from build123d import *

# Parameters (mm, degrees)
SKETCH1_W               = 20
SKETCH1_H               = 20
BOSS_EXTRUDE1_DEPTH     = 5
SKETCH2_W               = 20
SKETCH2_H               = 3
BOSS_EXTRUDE2_DEPTH     = 20
CUT_EXTRUDE1_DEPTH      = 25.494897428
CUT_EXTRUDE1_DEPTH_BACK = 25.494897428
SKETCH3_R               = 2.6
BOSS_EXTRUDE3_DEPTH     = 2
BOSS_EXTRUDE4_DEPTH     = 2
SKETCH6_W               = 2
SKETCH6_H               = 3
SKETCH6_W_2             = 4
BOSS_EXTRUDE5_DEPTH     = 0.8
SKETCH9_W               = 20
SKETCH9_H               = 3
BOSS_EXTRUDE8_DEPTH     = 45
BOSS_EXTRUDE9_DEPTH     = 20
SKETCH13_W              = 20
SKETCH13_H              = 3
BOSS_EXTRUDE12_DEPTH    = 80
SKETCH16_W              = 3
SKETCH16_H              = 45
CUT_EXTRUDE3_DEPTH      = 80
SKETCH22_W              = 20
SKETCH22_H              = 80
BOSS_EXTRUDE15_DEPTH    = 3
BOSS_EXTRUDE16_DEPTH    = 2
BOSS_EXTRUDE17_DEPTH    = 2
FILLET2_R               = 3
SKETCH26_R              = 2.4
CUT_EXTRUDE5_DEPTH      = 9


with BuildPart() as part:
    # Sketch1 → Boss-Extrude1 (new body)
    with BuildSketch(Plane(origin=(0, 0, 0), x_dir=(1, 0, 0), z_dir=(0, 1, 0))):
        Rectangle(SKETCH1_W, SKETCH1_H)
    extrude(amount=BOSS_EXTRUDE1_DEPTH)

    # Sketch2 → Boss-Extrude2 (add)
    with BuildSketch(Plane(origin=(0, 5, 0), x_dir=(1, 0, 0), z_dir=(0, 1, 0))):
        with Locations((0, 8.5)):
            Rectangle(SKETCH2_W, SKETCH2_H)
    extrude(amount=BOSS_EXTRUDE2_DEPTH)

    # Sketch3 → Cut-Extrude1 (cut, two sides: drawn at the far end of the back side and taken through both)
    with BuildSketch(Plane(origin=(0, 5, 0), x_dir=(1, 0, 0), z_dir=(0, 1, 0)).offset(-CUT_EXTRUDE1_DEPTH_BACK)):
        with Locations(Location((0, -1.5, 0), (0, 0, 270))):
            Circle(SKETCH3_R)
    extrude(amount=CUT_EXTRUDE1_DEPTH + CUT_EXTRUDE1_DEPTH_BACK, mode=Mode.SUBTRACT)

    # Sketch4 → Boss-Extrude3 (add)
    with BuildSketch(Plane.ZY.offset(10)):
        Polygon((-7, 25), (10, 5), (-7, 5), align=None)
    extrude(amount=-BOSS_EXTRUDE3_DEPTH)

    # Sketch5 → Boss-Extrude4 (add)
    with BuildSketch(Plane(origin=(10, 0, 0), x_dir=(0, 0, -1), z_dir=(1, 0, 0))):
        Polygon((7, 25), (-10, 5), (7, 5), align=None)
    extrude(amount=-BOSS_EXTRUDE4_DEPTH)

    # Sketch6 → Boss-Extrude5 (add)
    with BuildSketch(Plane(origin=(0, 0, 0), x_dir=(-1, 0, 0), z_dir=(0, -1, 0))):
        with Locations((-1, 4.297300947)):
            Rectangle(SKETCH6_W, SKETCH6_H)
        with Locations((1, 4.297300947)):
            Rectangle(SKETCH6_W, SKETCH6_H)
        with Locations((0, -7.297300947)):
            Rectangle(SKETCH6_W_2, SKETCH6_H)
    extrude(amount=BOSS_EXTRUDE5_DEPTH)

    # Sketch9 → Boss-Extrude8 (add)
    with BuildSketch(Plane(origin=(0, 25, 0), x_dir=(1, 0, 0), z_dir=(0, 1, 0))):
        with Locations((0, 8.5)):
            Rectangle(SKETCH9_W, SKETCH9_H)
    extrude(amount=BOSS_EXTRUDE8_DEPTH)

    # Sketch12 → Boss-Extrude9 (add)
    with BuildSketch(Plane(origin=(0, 0, -10), x_dir=(-1, 0, 0), z_dir=(0, 0, -1))):
        Polygon((0, 10), (-10, 10), (-10, 15), (10, 15), (10, 10), align=None)
    extrude(amount=BOSS_EXTRUDE9_DEPTH)

    # Sketch13 → Boss-Extrude12 (add)
    with BuildSketch(Plane(origin=(0, 15, 0), x_dir=(1, 0, 0), z_dir=(0, 1, 0))):
        with Locations((0, 28.5)):
            Rectangle(SKETCH13_W, SKETCH13_H)
    extrude(amount=BOSS_EXTRUDE12_DEPTH)

    # Sketch16 → Cut-Extrude3 (cut)
    with BuildSketch(Plane.ZY.offset(10)):
        with Locations((-8.5, 47.5)):
            Rectangle(SKETCH16_W, SKETCH16_H)
    extrude(amount=-CUT_EXTRUDE3_DEPTH, mode=Mode.SUBTRACT)

    # Sketch22 → Boss-Extrude15 (add)
    with BuildSketch(Plane.XY.offset(-27)):
        with Locations((0, 55)):
            Rectangle(SKETCH22_W, SKETCH22_H)
    extrude(amount=BOSS_EXTRUDE15_DEPTH)

    # Sketch23 → Boss-Extrude16 (add)
    with BuildSketch(Plane.ZY.offset(10)):
        Polygon((-24, 95), (-10, 25), (-10, 15), (-24, 15), align=None)
    extrude(amount=-BOSS_EXTRUDE16_DEPTH)

    # Sketch24 → Boss-Extrude17 (add)
    with BuildSketch(Plane(origin=(10, 0, 0), x_dir=(0, 0, -1), z_dir=(1, 0, 0))):
        Polygon((24, 95), (10, 25), (10, 15), (24, 15), align=None)
    extrude(amount=-BOSS_EXTRUDE17_DEPTH)

    # Fillet2
    # the kernel refuses this fillet: 3 mm, written as the material it takes off along each edge
    with BuildSketch(Plane(origin=(-10, 95, -16.5), x_dir=(0, -1, 0), z_dir=(0, 0, -1)), Plane(origin=(10, 95, -37.5), x_dir=(0, -1, 0), z_dir=(0, 0, 1))) as fillet2_piece_1:
        with BuildLine():
            CenterArc((FILLET2_R, -FILLET2_R), FILLET2_R, 90, 90)
            Line((0, -FILLET2_R), (0, 0))
            Line((0, 0), (FILLET2_R, 0))
        make_face()
    extrude(amount=21, mode=Mode.SUBTRACT)

    # Sketch26 → Cut-Extrude5 (cut)
    with BuildSketch(Plane(origin=(0, 0, -30), x_dir=(-1, 0, 0), z_dir=(0, 0, -1))):
        with Locations((-0.179346542, 85.282473515)):
            Circle(SKETCH26_R)
        with Locations((-0.179346542, 20.282473515)):
            Circle(SKETCH26_R)
    extrude(amount=-CUT_EXTRUDE5_DEPTH, mode=Mode.SUBTRACT)


solid = part.part
Model file for the job. Use its own axes, mm. A direction names the side the tool comes from. Coordinates: 2 decimals unless noted, no trailing zeros. Order: outer loops, then holes, each group sorted by start corner. A loop starts at its lowest first (then second) coordinate and runs counter-clockwise, first axis right, second up. Notation, with made-up numbers: (-11, 86.25) -> (11, 86.25) arc R6 cw to (11, 96.25) -> close; hole circle Ø7 at (69, -18.5). An arc over 180 degrees is marked (long way). Return JSON: item names as keys, results as strings. Group by question number.
Item 1: Flat gauge pins, fed straight in: P1, Ø4, axis at y = 74.5, z = -17, coming from the -X side; P2, Ø0.9, axis at y = -0.5, z = -4.5, coming from the +X side; P3, Ø5, axis at x = -2.5, y = 49.5, coming from the +Z side; P4, Ø6, axis at x = 3.5, z = -1, coming from the +Y side. Where does each tip first touch, or does it go through?
Item 2: Tool access for faces 1 (the flat face through (-8, 11, -2)), 2 (the cylindrical face through (0.7, 17.94, -27.04)), 3 (the flat face through (0, 25, -9)): list every direction of +Z, -Z, +X, -X, +Y, -Y with a clear straight run to the whole face (end or side of a thin tool).
Item 3: Saw through at A-A on z = 1.5. Write the cut outline in (x, y).
Item 4: Wall check: line 1 along X through (y, z) = (3.55, 1.5); line 2 along X through (y, z) = (52, -20.5); line 3 along Z through (x, y) = (2.5, 16). Give the ranges that are in metal, low to high. Write a range as [from, to].
Item 5: Saw through at C-C on x = 0. State how many separate pieces and enclosed holes the cut face has, then the cut area to 3 significant figures.
Item 6: Pull direction Z, two halves, no side cores. Call faces 4 (the flat face through (0, 15, -17)), 5 (the flat face through (0, 2, 10)), 6 (the flat face through (-8, 47, -18)), 7 (the flat face through (0, -0.8, -4)): pulls with the +Z half, pulls with the -Z half, needs draft (parallel to the pull), parting line crosses it, or undercut.
Item 7: Saw through at B-B on y = 66.5. Write the cut outline in (x, z), then the cut area to 3 significant figures.
Item 8: Saw through at D-D on z = -20. Write the cut outline in (x, y).
Values found:
{
 "1": {"P1": "passes through", "P2": "stops at x = 2", "P3": "stops at z = -24", "P4": "stops at y = 5"},
 "2": {"face 1": "+Z, +Y", "face 2": "-Z", "face 3": "+Z, +X, -X, +Y"},
 "3": {"outline": "(-10, 0) -> (-2.6, 0) -> (-2.6, 5) -> (-8, 5) -> (-8, 15) -> (-10, 15) -> close; (2.6, 0) -> (10, 0) -> (10, 15) -> (8, 15) -> (8, 5) -> (2.6, 5) -> close"},
 "4": {"line 1": "x = [-10, -2.6], [2.6, 10]", "line 2": "x = [-10, -8], [8, 10]", "line 3": "z = [-30, -24], [-10, -7]"},
 "5": {"separate pieces": "4", "enclosed holes": "0", "area": "661 mm2"},
 "6": {"face 4": "undercut", "face 5": "pulls with the +Z half", "face 6": "undercut", "face 7": "needs draft"},
 "7": {"outline": "(-10, -30) -> (10, -30) -> (10, -18.3) -> (8, -18.3) -> (8, -24) -> (-8, -24) -> (-8, -18.3) -> (-10, -18.3) -> close", "area": "143 mm2"},
 "8": {"outline": "(-10, 10) -> (10, 10) -> (10, 75) -> (8, 75) -> (8, 15) -> (-8, 15) -> (-8, 75) -> (-10, 75) -> close"}
}
